Input: part model. Units: mm. Frame: model coordinates. A direction names the side the tool comes from. Coordinates: 2 decimals unless noted, no trailing zeros. Order: outer loops, then holes, each group sorted by start corner. A loop starts at its lowest first (then second) coordinate and runs counter-clockwise, first axis right, second up. Notation, with made-up numbers: M 15,88.5 L 20,88.5 A14 ccw 20,115.5 Z; hole C -14.75,-9.5 d11. An arc over 180 degrees is marked long. Answer in a Markdown table with one row per item.
from build123d import *

# Parameters (mm, degrees)
SKETCH1_W           = 77
SKETCH1_H           = 45
BOSS_EXTRUDE1_DEPTH = 2
SKETCH2_W           = 77
SKETCH2_H           = 45
SKETCH2_W_2         = 73
SKETCH2_H_2         = 41
BOSS_EXTRUDE2_DEPTH = 20
SKETCH3_W           = 2
SKETCH3_H           = 45
BOSS_EXTRUDE3_DEPTH = 29
SKETCH4_R           = 1.25
CUT_EXTRUDE1_DEPTH  = 2
SKETCH5_R           = 1.25
CUT_EXTRUDE2_DEPTH  = 2
SKETCH6_W           = 9.5
SKETCH6_H           = 11.1
CUT_EXTRUDE3_DEPTH  = 2
SKETCH7_W           = 8.5
SKETCH7_H           = 3.5
CUT_EXTRUDE4_DEPTH  = 2
SKETCH8_W           = 4
SKETCH8_H           = 4
CUT_EXTRUDE5_DEPTH  = 2


with BuildPart() as part:
    # Sketch1 → Boss-Extrude1 (new body)
    with BuildSketch(Plane(origin=(0, 0, 0), x_dir=(1, 0, 0), z_dir=(0, 1, 0))):
        Rectangle(SKETCH1_W, SKETCH1_H)
    extrude(amount=BOSS_EXTRUDE1_DEPTH)

    # Sketch2 → Boss-Extrude2 (add)
    with BuildSketch(Plane(origin=(0, 2, 0), x_dir=(1, 0, 0), z_dir=(0, 1, 0))):
        Rectangle(SKETCH2_W, SKETCH2_H)
        Rectangle(SKETCH2_W_2, SKETCH2_H_2, mode=Mode.SUBTRACT)
    extrude(amount=BOSS_EXTRUDE2_DEPTH)

    # Sketch3 → Boss-Extrude3 (add)
    with BuildSketch(Plane(origin=(0, 22, 0), x_dir=(1, 0, 0), z_dir=(0, 1, 0))):
        with Locations((-37.5, 0)):
            Rectangle(SKETCH3_W, SKETCH3_H)
    extrude(amount=BOSS_EXTRUDE3_DEPTH)

    # Sketch4 → Cut-Extrude1 (cut)
    with BuildSketch(Plane(origin=(0, 0, -22.5), x_dir=(-1, 0, 0), z_dir=(0, 0, -1))):
        with Locations((-32.5, 18)):
            Circle(SKETCH4_R)
    extrude(amount=-CUT_EXTRUDE1_DEPTH, mode=Mode.SUBTRACT)

    # Sketch5 → Cut-Extrude2 (cut)
    with BuildSketch(Plane.XY.offset(22.5)):
        with Locations((-30.5, 18)):
            Circle(SKETCH5_R)
    extrude(amount=-CUT_EXTRUDE2_DEPTH, mode=Mode.SUBTRACT)

    # Sketch6 → Cut-Extrude3 (cut)
    with BuildSketch(Plane.XY.offset(22.5)):
        with Locations((-14.52, 16.45)):
            Rectangle(SKETCH6_W, SKETCH6_H)
    extrude(amount=-CUT_EXTRUDE3_DEPTH, mode=Mode.SUBTRACT)

    # Sketch7 → Cut-Extrude4 (cut)
    with BuildSketch(Plane(origin=(0, 0, -22.5), x_dir=(-1, 0, 0), z_dir=(0, 0, -1))):
        with Locations((7.62, 20.25)):
            Rectangle(SKETCH7_W, SKETCH7_H)
    extrude(amount=-CUT_EXTRUDE4_DEPTH, mode=Mode.SUBTRACT)

    # Sketch8 → Cut-Extrude5 (cut)
    with BuildSketch(Plane(origin=(38.5, 0, 0), x_dir=(0, 0, -1), z_dir=(1, 0, 0))):
        with Locations((0, 20)):
            Rectangle(SKETCH8_W, SKETCH8_H)
    extrude(amount=-CUT_EXTRUDE5_DEPTH, mode=Mode.SUBTRACT)


solid = part.part
1) Cut plane B-B, the plane z = -4.5. Output: boundary loops of the cut face in (x, y), and give its area (3 significant figures).
Resolved:
| item | result |
|---|---|
| outline | M -38.5,0 L 38.5,0 L 38.5,22 L 36.5,22 L 36.5,2 L -36.5,2 L -36.5,51 L -38.5,51 Z |
| area | 292 mm2 |
2) Cut plane A-A, the plane x = 32.5. Output: boundary loops of the cut face in (y, z).
Resolved:
| item | result |
|---|---|
| outline | M 0,-22.5 L 16.75,-22.5 L 16.75,-20.5 L 2,-20.5 L 2,20.5 L 22,20.5 L 22,22.5 L 0,22.5 Z; M 19.25,-22.5 L 22,-22.5 L 22,-20.5 L 19.25,-20.5 Z |
3) Contact query for flat-ended pins moving along their axis: pin 1 (4 mm diameter, centred on x = -8, z = -6.5, fed in from +Y); pin 2 (1 mm diameter, centred on x = -8.5, z = -21.5, fed in from +Y); pin 3 (2 mm diameter, centred on x = -30.5, y = 18, fed in from +Z). Output: stop coordinate, or through.
Resolved:
| item | result |
|---|---|
| pin 1 | stops at y = 2 |
| pin 2 | stops at y = 18.5 |
| pin 3 | stops at z = -20.5 |
4) Mould query, pull axis Y, two halves, no side actions, for faces 6 (the face through (-1, 0, 0)), 7 (the face through (-36.5, 26, 0)), 8 (the face through (-24, 22, -22)), 9 (the face through (31.345, 17.521, -21.514)). Classes: +Y half, -Y half, draft (parallel to the pull), parting line (faces both ways), or undercut.
Resolved:
| item | result |
|---|---|
| face 6 | -Y half |
| face 7 | draft |
| face 8 | +Y half |
| face 9 | undercut |
5) Cut plane C-C, the plane y = 3.5. Output: boundary loops of the cut face in (x, z), and give its area (3 significant figures).
Resolved:
| item | result |
|---|---|
| outline | M -38.5,-22.5 L 38.5,-22.5 L 38.5,22.5 L -38.5,22.5 Z; hole M -36.5,-20.5 L 36.5,-20.5 L 36.5,20.5 L -36.5,20.5 Z |
| area | 472 mm2 |
6) Material intervals for probe 1 along Z at (x, y) = (19.5, 21); probe 2 along Y at (x, z) = (32.5, -22); probe 3 along X at (y, z) = (7, -16.5), sorted ascending.
Resolved:
| item | result |
|---|---|
| probe 1 | z = -22.5 to -20.5, 20.5 to 22.5 |
| probe 2 | y = 0 to 16.75, 19.25 to 22 |
| probe 3 | x = -38.5 to -36.5, 36.5 to 38.5 |
7) Cut plane D-D, the plane x = 14. Output: boundary loops of the cut face in (y, z).
Resolved:
| item | result |
|---|---|
| outline | M 0,-22.5 L 22,-22.5 L 22,-20.5 L 2,-20.5 L 2,20.5 L 22,20.5 L 22,22.5 L 0,22.5 Z |
8) Reachability of faces 1 (the face through (36.5, 12, 0)), 2 (the face through (21, 22, -21)), 3 (the face through (-19.27, 16, 22)), 4 (the face through (-8, 18.5, -22)), 5 (the face through (38, 18, 0)) from +Z, -Z, +X, -X, +Y, -Y: full face, straight path, thin tool, end or side. Return the list, or none.
Resolved:
| item | result |
|---|---|
| face 1 | +Y |
| face 2 | +Z, -Z, +X, +Y |
| face 3 | +Z, +Y |
| face 4 | -Z, +Y |
| face 5 | +X, +Y |
